The drawing under review shows one solid part. Ordinate dimensions are in mm from its lowest x, y, z. A direction names the side the tool comes from. Round coordinates to 2 decimals unless told otherwise and drop trailing zeros. Write each loop counter-clockwise with the first axis right and the second up, starting at its lowest first coordinate (ties: lowest second). Pieces come first, ordered by that corner, then holes. Notation, with made-up numbers: (69, 61) -> (83, 61) arc R20 ccw to (83, 66) -> close; hole circle Ø4 at (15.5, -19). An arc over 180 degrees is marked (long way). Write item = value, one per line. Start each with the question number.
Item 1: Add section B-B, the plane y = 317.5. State the section outline as (x, z) points, then the cut area to 3 significant figures.
Item 2: Add section A-A, the plane x = 266.7. State the section outline as (y, z) points.
Item 3: To check wall thickness, follow L1, parallel to Y at x = 397, z = 773.5; L2, parallel to Z at x = 325.5, y = 304; L3, parallel to Z at x = 101.5, y = 234. State the ranges of each line that lie inside material, in increasing order.
Item 4: For pin 1 Ø4 at (x, z) = (163, 684) entering from -Y; pin 2 Ø1.5 at (x, z) = (276.5, 231.5) entering from +Y; pin 3 Ø6 at (x, y) = (364, 493) entering from +Z; pin 4 Ø8 at (x, y) = (372, 108) entering from -Z, all flat-tipped, find the tip position at first contact; note any pin that passes through.
Item 5: Add section D-D, the plane x = 324. State the section outline as (y, z) points, then the cut area to 3 significant figures.
Item 6: Machinability: for the marked faces 1, 2 and 3, which of the approach directions +Z, -Z, +X, -X, +Y, -Y give a long, thin tool a straight path to every point of the face, cutting with its end or side? Answer none if there is none.
Item 7: Add section C-C, the plane z = 354. State the section outline as (x, y) points, then the cut area to 3 significant figures.
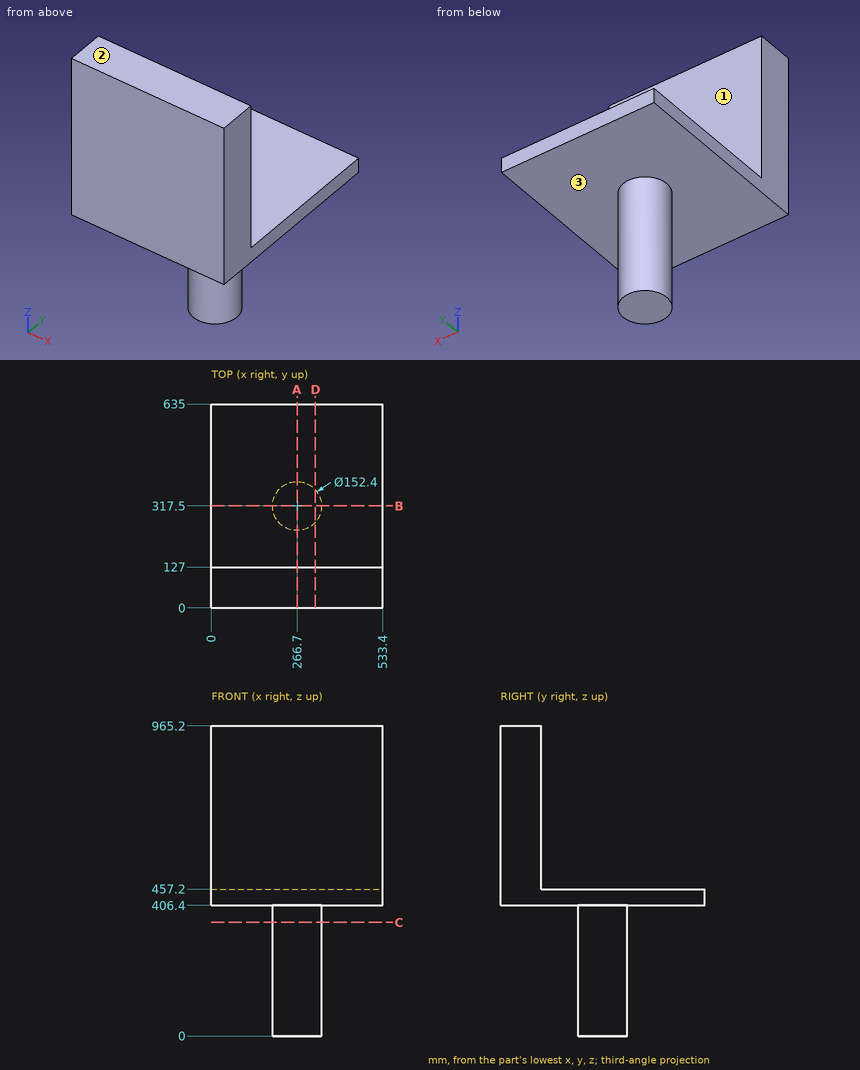
Result set:
q1.outline = (0, 406.4) -> (190.5, 406.4) -> (190.5, 0) -> (342.9, 0) -> (342.9, 406.4) -> (533.4, 406.4) -> (533.4, 457.2) -> (0, 457.2) -> close
q1.area = 89,000 mm²
q2.outline = (0, 406.4) -> (241.3, 406.4) -> (241.3, 0) -> (393.7, 0) -> (393.7, 406.4) -> (635, 406.4) -> (635, 457.2) -> (127, 457.2) -> (127, 965.2) -> (0, 965.2) -> close
q3.L1 = 0 to 127
q3.L2 = 0 to 457.2
q3.L3 = 406.4 to 457.2
q4.pin_1 = 0
q4.pin_2 = 393.16
q4.pin_3 = 457.2
q4.pin_4 = 406.4
q5.outline = (0, 406.4) -> (267.27, 406.4) -> (267.27, 0) -> (367.73, 0) -> (367.73, 406.4) -> (635, 406.4) -> (635, 457.2) -> (127, 457.2) -> (127, 965.2) -> (0, 965.2) -> close
q5.area = 138,000 mm²
q6.face_1 = +Z, +X, -X, +Y
q6.face_2 = +Z, +X, -X, +Y, -Y
q6.face_3 = -Z
q7.outline = circle Ø152.4 at (266.7, 317.5)
q7.area = 18,200 mm²
